Can you work these out from the model? Positions are in its coordinate system, mm. Round coordinates to 2 decimals unless told otherwise and drop trailing zeros. Loops run counter-clockwise (first coordinate to the right, second up) from the corner with the lowest first, then second, coordinate; pieces in that order, holes last.
from build123d import *

# Parameters (mm, degrees)
ESQUISSE1_W             = 2000
ESQUISSE1_H             = 1000
BOSS_EXTRU_1_DEPTH      = 300
CHANFREIN1_SIZE         = 100
ESQUISSE2_R             = 75
ESQUISSE2_R_2           = 225
ESQUISSE2_R_3           = 150
ENL_V_MAT_EXTRU_1_DEPTH = 1158.583690279
CHANFREIN2_SIZE         = 50


with BuildPart() as part:
    # Esquisse1 → Boss.-Extru.1 (new body)
    with BuildSketch(Plane.XY):
        Rectangle(ESQUISSE1_W, ESQUISSE1_H)
    extrude(amount=BOSS_EXTRU_1_DEPTH)

    # Chanfrein1
    chanfrein1_edges = [part.edges().sort_by_distance(p)[0] for p in [
        (-1000, 0, 300),
        (0, -500, 300),
        (1000, 0, 300),
        (0, -500, 0),
        (-1000, 0, 0),
        (0, 500, 0),
        (1000, 0, 0),
        (0, 500, 300),
    ]]
    chamfer(chanfrein1_edges, length=CHANFREIN1_SIZE)

    # Esquisse2 → Enlèv. mat.-Extru.1 (cut, through all)
    with BuildSketch(Plane(origin=(0, 0, 0), x_dir=(-1, 0, 0), z_dir=(0, 0, -1))):
        with Locations((-750, 0)):
            Circle(ESQUISSE2_R)
        with Locations((500, 0)):
            Circle(ESQUISSE2_R_2)
        with Locations((-250, 0)):
            Circle(ESQUISSE2_R_3)
    extrude(amount=-ENL_V_MAT_EXTRU_1_DEPTH, mode=Mode.SUBTRACT)

    # Chanfrein2
    chanfrein2_edges = [part.edges().sort_by_distance(p)[0] for p in [
        (825, 0, 0),
        (400, 0, 0),
        (-275, 0, 0),
    ]]
    chamfer(chanfrein2_edges, length=CHANFREIN2_SIZE)


solid = part.part
(1) If we section it at A-A, the plane z = 281: List the corners of the cut face in (x, y) for me.
Worked answers:
outline: (-919, -419) - (919, -419) - (919, 419) - (-919, 419) - close; hole circle Ø450 at (-500, 0); hole circle Ø300 at (250, 0); hole circle Ø150 at (750, 0)
(2) Will these pins go through, and if not, where does the flat tip stop? P1, Ø5, axis at x = -570, z = 32.5, coming from the +Y side; P2, Ø10, axis at y = -364, z = 259, coming from the -X side; P3, Ø5, axis at y = 345, z = 216, coming from the +X side.
Worked answers:
P1: stops at y = 435
P2: stops at x = -946
P3: stops at x = 986.5
(3) If we mould it in two halves opening along X, with no side actions, what happens to faces 1 (the cylindrical face through (809.517, -45.636, 173.25)), 2 (the flat face through (-14, 449, 49)), 3 (the flat face through (1000, -7, 149))? For each: released by +X, released by -X, zero draft, split by the parting line, or undercut.
Worked answers:
face 1: undercut
face 2: zero draft
face 3: released by +X
(4) If we section it at D-D, the plane y = 313: List the corners of the cut face in (x, z) for me, then the cut area to 3 significant figures.
Worked answers:
outline: (-1000, 100) - (-900, 0) - (900, 0) - (1000, 100) - (1000, 200) - (900, 300) - (-900, 300) - (-1000, 200) - close
area: 580,000 mm2
(5) If we section it at C-C, the plane y = 0: List the corners of the cut face in (x, z) for me, then the cut area to 4 significant figures.
Worked answers:
outline: (-1000, 100) - (-900, 0) - (-775, 0) - (-725, 50) - (-725, 300) - (-900, 300) - (-1000, 200) - close; (-275, 50) - (-225, 0) - (50, 0) - (100, 50) - (100, 300) - (-275, 300) - close; (400, 50) - (450, 0) - (625, 0) - (675, 50) - (675, 300) - (400, 300) - close; (825, 50) - (875, 0) - (900, 0) - (1000, 100) - (1000, 200) - (900, 300) - (825, 300) - close
area: 302,500 mm2
(6) If I drill on line 1 (Y direction, x = -487, z = 198.5); line 2 (X direction, y = -50.5, z = 253); line 3 (X direction, y = -64, z = 238), over which ranges is the centre line in solid material (lowest first)?
Worked answers:
line 1: y = -500 to -224.62, 224.62 to 500
line 2: x = -947 to -719.26, -280.74 to 108.76, 391.24 to 694.55, 805.45 to 947
line 3: x = -962 to -715.71, -284.29 to 114.34, 385.66 to 710.9, 789.1 to 962
(7) If we section it at B-B, the plane x = 250: List the corners of the cut face in (y, z) for me, then the cut area to 4 significant figures.
Worked answers:
outline: (-500, 100) - (-400, 0) - (-200, 0) - (-150, 50) - (-150, 300) - (-400, 300) - (-500, 200) - close; (150, 50) - (200, 0) - (400, 0) - (500, 100) - (500, 200) - (400, 300) - (150, 300) - close
area: 187,500 mm2
